```python
from build123d import *

# Parameters (mm, degrees)
F0_W   = 26.1907838285
F0_H   = 4.2092371732
F0_W_2 = 7.9507762566
F0_W_3 = 3.7415362895
F0_W_4 = 12.6277022064
F0_W_5 = 12.6276984811
F0_W_6 = 49.1077229381
F0_W_7 = 14.0307797119


# Not quite as in the source:
# - ends of sketch curves that miss each other by under 0.0002 mm in the source are joined
# - the program builds the solid bodies; features that only make, move or delete a surface that nothing else refers to are left out


with BuildPart() as f1:
    # F0 (on Front) → F1 (revolve)
    with BuildSketch(Plane.XZ):
        with Locations((-35.0769478828, 2.1046185866)):
            Rectangle(F0_W, F0_H)
        with Locations((-3.9753881283, 2.1046185866)):
            Rectangle(F0_W_2, F0_H)
        with Locations((-62.6708101481, 2.1046185866)):
            Rectangle(F0_W_3, F0_H)
        with Locations((-54.4861909002, 2.1046185866)):
            Rectangle(F0_W_4, F0_H)
        with Locations((-70.8554275334, 2.1046185866)):
            Rectangle(F0_W_5, F0_H)
        with Locations((-101.723138243, 2.1046185866)):
            Rectangle(F0_W_6, F0_H)
        Polygon((-21.9815559685, 44.8984950781), (-21.9815559685, 4.2092371732), (-7.9507762566, 4.2092371732), (-7.9507762566, 44.8984950781), (-12.1600097045, 44.8984950781), (-12.1600097045, 37.4154113233), (-17.3046290874, 37.4154113233), (-17.3046290874, 44.8984950781), align=None)
        with Locations((-14.9661661126, 2.1046185866)):
            Rectangle(F0_W_7, F0_H)
        Polygon((-60.8000420034, 27.1261744201), (-60.8000420034, 4.2092371732), (-48.172339797, 4.2092371732), (-48.172339797, 27.1261744201), (-52.8492666781, 27.1261744201), (-52.8492666781, 21.0461709648), (-56.5908066928, 21.0461709648), (-56.5908066928, 27.1261744201), align=None)
        Polygon((-77.1692767739, 27.1261744201), (-77.1692767739, 4.2092371732), (-64.5415782928, 4.2092371732), (-64.5415782928, 27.1261744201), (-68.7508136034, 27.1261744201), (-68.7508136034, 21.0461709648), (-72.960048914, 21.0461709648), (-72.960048914, 27.1261744201), align=None)
        Polygon((-139.37240839, 27.1261744201), (-139.37240839, 0), (-126.276999712, 0), (-126.276999712, 4.2092371732), (-126.276999712, 27.1261744201), (-130.4862499237, 27.1261744201), (-130.4862499237, 21.0461709648), (-134.6954703331, 21.0461709648), (-134.6954703331, 27.1261744201), align=None)
        Polygon((0, 4.2092371732), (0, 0), (35.0769385695, 0), (35.0769385695, 37.4154113233), (31.3354022801, 37.4154113233), (31.3354022801, 41.1569550633), (18.7077019364, 50.9784966707), (18.7077019364, 57.993888855), (12.1600031853, 57.993888855), (12.1600031853, 50.9784966707), (6.080001127, 50.9784966707), (6.080001127, 57.993888855), (-1.2167e-06, 57.993888855), align=None)
        Polygon((35.0769385695, 37.4154113233), (35.0769385695, 0), (65.9446567297, 0), (65.9446567297, 50.9784966707), (65.9446567297, 57.993888855), (59.396956116, 57.993888855), (59.396956116, 50.9784966707), (55.187728256, 50.9784966707), (55.187728256, 57.993888855), (47.7046445012, 57.993888855), (47.7046445012, 50.9784966707), (35.0769385695, 41.1569550633), align=None)
    revolve(axis=Axis((-53.7846479565, 0, -3.7415372208), (1, 0, 0)))


solid = f1.part
```
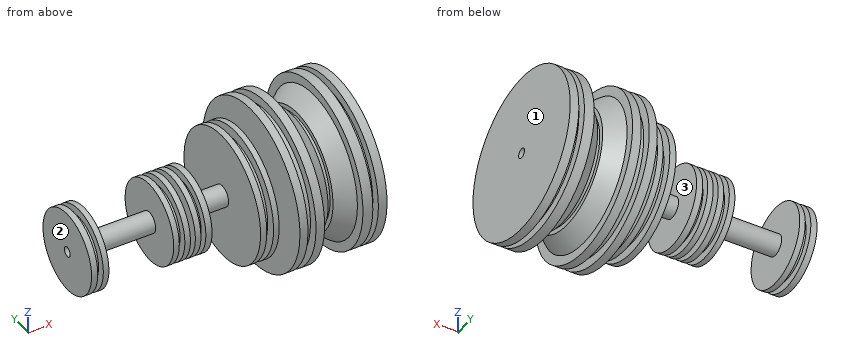
Check sheet for the modelled part. Datum: model origin and axes. Units: mm. Face numbers are marked on the shaded views. Round coordinates to 2 decimals unless told otherwise and drop trailing zeros. Order: outer loops, then holes, each group sorted by start corner. A loop starts at its lowest first (then second) coordinate and runs counter-clockwise, first axis right, second up.
1) Go/stop test with flat-tipped pins: pin 1 Ø2 at (y, z) = (-3.5, -37) entering from -X; pin 2 Ø6 at (x, z) = (39, -27.5) entering from +Y; pin 3 Ø8 at (y, z) = (-37.5, 40) entering from -X. Record where each tip stops, or that it passes through.
2) Section check B-B (y = 15). Give the number of separate pieces and of enclosed holes in the cut face, and give its area (3 significant figures).
3) Scan lines: line 1 (X direction, y = -1, z = -21); line 2 (X direction, y = -32, z = 5); line 3 (X direction, y = -3.5, z = -45). Record each from-to range of solid material in increasing order.
4) Section check A-A (x = -34.5). Record the boundary of the cut face in (y, z).
5) Mould release check, pull along X, two halves, no side actions. Record for the marked faces 1, 2 and 3: +X half, -X half, draft (parallel to the pull), parting line (faces both ways), or undercut.
Result:
1. pin 1: stops at x = -21.98
1. pin 2: stops at y = 44.74
1. pin 3: stops at x = 0
2. separate pieces: 5
2. enclosed holes: 0
2. area: 10,100 mm2
3. line 1: x = -139.37 to -126.28, -77.17 to -64.54, -60.8 to -48.17, -21.98 to -7.95, 0 to 65.94
3. line 2: x = -21.98 to -7.95, 0 to 65.94
3. line 3: x = -21.98 to -17.3, -12.16 to -7.95, 0 to 31.34, 35.08 to 65.94
4. outline: circle Ø15.9 at (0, -3.74); hole circle Ø7.48 at (0, -3.74)
5. face 1: +X half
5. face 2: -X half
5. face 3: undercut
